Build history of the part. All positions in model axes, mm. A direction names the side the tool comes from. Give positions to 0.01 mm unless a question says otherwise; leave off trailing zeros. Write each loop counter-clockwise with the first axis right and the second up, starting at its lowest first coordinate (ties: lowest second). Pieces come first, ordered by that corner, then holes. Notation, with made-up numbers: (78, -23) - (117, -23) arc R17 cw to (117, 0) - close; hole circle Ø2 at (-29, 15.25). An arc over 180 degrees is marked (long way). Use one line per item in the form item = value. Start each with the question number.
from build123d import *

# Parameters (mm, degrees)
BOSS_EXTRUDE1_DEPTH = 231.201214
BOSS_EXTRUDE2_START = -12.852654
BOSS_EXTRUDE2_DEPTH = 6.35
SKETCH3_R           = 15.942437
CUT_EXTRUDE1_DEPTH  = 842.74192987


with BuildPart() as part:
    # Sketch1 → Boss-Extrude1 (new body)
    with BuildSketch(Plane.XY):
        with BuildLine():
            Line((-90.736928, 597.708228), (90.721434, 597.708228))
            ThreePointArc((90.721434, 597.708228), (103.921108752, 602.235738137), (111.562896, 613.911904))
            Line((111.562896, 613.911904), (111.562896, 761.795784))
            ThreePointArc((111.562896, 761.795784), (103.921186704, 773.472121096), (90.721434, 777.999714))
            Line((90.721434, 777.999714), (-90.736928, 777.999714))
            ThreePointArc((-90.736928, 777.999714), (-103.936580442, 773.472111924), (-111.578136, 761.795784))
            Line((-111.578136, 761.795784), (-111.578136, 613.911904))
            ThreePointArc((-111.578136, 613.911904), (-103.936502489, 602.235747309), (-90.736928, 597.708228))
        make_face()
        with BuildLine():
            Line((-90.736928, 604.150176), (90.721434, 604.150176))
            ThreePointArc((90.721434, 604.150176), (99.673810429, 607.099124575), (105.120948, 614.791330612))
            Line((105.120948, 614.791330612), (105.120948, 760.91641141))
            ThreePointArc((105.120948, 760.91641141), (99.673869855, 768.60875328), (90.721434, 771.557766))
            Line((90.721434, 771.557766), (-90.736928, 771.557766))
            ThreePointArc((-90.736928, 771.557766), (-99.689249554, 768.60875822), (-105.136188, 760.916452346))
            Line((-105.136188, 760.916452346), (-105.136188, 614.791289676))
            ThreePointArc((-105.136188, 614.791289676), (-99.689190128, 607.099119635), (-90.736928, 604.150176))
        make_face(mode=Mode.SUBTRACT)
    extrude(amount=-BOSS_EXTRUDE1_DEPTH)

    # Sketch1_2 → Boss-Extrude2 (add)
    with BuildSketch(Plane.XY.offset(BOSS_EXTRUDE2_START)):
        with BuildLine():
            ThreePointArc((-90.736928, 604.150176), (-99.689190128, 607.099119635), (-105.136188, 614.791289676))
            Line((-105.136188, 614.791289676), (-105.136188, 760.916452346))
            ThreePointArc((-105.136188, 760.916452346), (-99.689249554, 768.60875822), (-90.736928, 771.557766))
            Line((-90.736928, 771.557766), (90.721434, 771.557766))
            ThreePointArc((90.721434, 771.557766), (99.673869855, 768.60875328), (105.120948, 760.91641141))
            Line((105.120948, 760.91641141), (105.120948, 614.791330612))
            ThreePointArc((105.120948, 614.791330612), (99.673810429, 607.099124575), (90.721434, 604.150176))
            Line((90.721434, 604.150176), (-90.736928, 604.150176))
        make_face()
        with BuildLine():
            Line((-90.736928, 604.150176), (-0.007747, 604.150176))
            Line((-0.007747, 604.150176), (-0.007747, 771.557766))
            Line((-0.007747, 771.557766), (-90.736928, 771.557766))
            ThreePointArc((-90.736928, 771.557766), (-99.689249554, 768.60875822), (-105.136188, 760.916452346))
            Line((-105.136188, 760.916452346), (-105.136188, 614.791289676))
            ThreePointArc((-105.136188, 614.791289676), (-99.689190128, 607.099119635), (-90.736928, 604.150176))
        make_face()
    extrude(amount=-BOSS_EXTRUDE2_DEPTH)

    # Sketch3 → Cut-Extrude1 (cut, through all)
    with BuildSketch(Plane(origin=(111.562896, 0, 0), x_dir=(0, 0, -1), z_dir=(1, 0, 0))):
        with Locations((170.56862, 661.318972)):
            Circle(SKETCH3_R)
    extrude(amount=-CUT_EXTRUDE1_DEPTH, mode=Mode.SUBTRACT)


solid = part.part
(1) Wall check: line 1 (Y direction, x = 0, z = -220.5); line 2 (X direction, y = 696, z = -165); line 3 (Z direction, x = -61, y = 701). Give the ranges that are in metal, low to high. Write a range as from..to.
(2) Which spindle directions (+Z, -Z, +X, -X, +Y, -Y) get a long thin tool onto all of the face, cutting with end or side? Do faces 1 (the flat face through (1, 778, -114)), 2 (the flat face through (1, 689, -12.853)), 3 (the cylindrical face through (99.566, 607.02, -123.718)). Say none if no direction does.
(3) Cut at C-C, the plane x = -39. Give the cut face in (y, z).
(4) Cut at B-B, the plane y = 742.5. Give the cut face in (x, z), then the cut area to 3 significant figures.
(5) Cut at A-A, the plane z = -204. Give the cut face in (x, y).
(6) Pin check, flat tip, straight feed: pin 1 Ø8 at (x, y) = (-63.5, 709) entering from -Z. Stop position of the tip, or through.
(7) Two-plate mould, pull along X, no slides. Class faces 4 (the cylindrical face through (-99.8, 607.18, -123.72)), 5 (the cylindrical face through (103.76, 602.11, -113.98)), 6 (the cylindrical face through (108.387, 677.126, -168.493)): +X half, -X half, draft (parallel to the pull), parting line (faces both ways), or undercut.
Solution:
q1.line_1 = 597.71..604.15, 771.56..778
q1.line_2 = -111.58..-105.14, 105.12..111.56
q1.line_3 = -19.2..-12.85
q2.face_1 = +Z, -Z, +X, -X, +Y
q2.face_2 = +Z
q2.face_3 = -Z
q3.outline = (597.71, -231.2) - (604.15, -231.2) - (604.15, -19.2) - (771.56, -19.2) - (771.56, -231.2) - (778, -231.2) - (778, 0) - (771.56, 0) - (771.56, -12.85) - (604.15, -12.85) - (604.15, 0) - (597.71, 0) - close
q4.outline = (-111.58, -231.2) - (-105.14, -231.2) - (-105.14, -19.2) - (105.12, -19.2) - (105.12, -231.2) - (111.56, -231.2) - (111.56, 0) - (105.12, 0) - (105.12, -12.85) - (-105.14, -12.85) - (-105.14, 0) - (-111.58, 0) - close
q4.area = 4,310 mm2
q5.outline = (-111.58, 613.91) arc R21.5 ccw to (-90.74, 597.71) - (90.72, 597.71) arc R21.51 ccw to (111.56, 613.91) - (111.56, 761.8) arc R21.51 ccw to (90.72, 778) - (-90.74, 778) arc R21.5 ccw to (-111.58, 761.8) - close; hole (-105.14, 614.79) arc R15.06 ccw to (-90.74, 604.15) - (90.72, 604.15) arc R15.06 ccw to (105.12, 614.79) - (105.12, 760.92) arc R15.06 ccw to (90.72, 771.56) - (-90.74, 771.56) arc R15.06 ccw to (-105.14, 760.92) - close
q6.pin_1 = -19.2
q7.face_4 = undercut
q7.face_5 = +X half
q7.face_6 = draft
